from build123d import *

# Parameters (mm, degrees)
SKETCH1_W           = 30
SKETCH1_H           = 75
BOSS_EXTRUDE1_DEPTH = 12
CUT_EXTRUDE1_DEPTH  = 12
LPATTERN1_COUNT     = 3
LPATTERN1_PITCH     = 20
CUT_EXTRUDE2_DEPTH  = 30
BOSS_EXTRUDE2_DEPTH = 30
BOUNDARY1_START     = -45
BOUNDARY1_DEPTH     = 5
LPATTERN2_COUNT     = 3
LPATTERN2_PITCH     = 20


# Read off the part's stored shape, not the designer's step: Boundary1
with BuildPart() as part:
    # Sketch1 → Boss-Extrude1 (new body)
    with BuildSketch(Plane(origin=(0, 0, 0), x_dir=(1, 0, 0), z_dir=(0, 1, 0))):
        with Locations((15, 37.5)):
            Rectangle(SKETCH1_W, SKETCH1_H)
    extrude(amount=BOSS_EXTRUDE1_DEPTH)

    # Sketch3 → Cut-Extrude1 (cut)
    with BuildSketch(Plane(origin=(0, 0, 0), x_dir=(1, 0, 0), z_dir=(0, 1, 0))):
        Polygon((0, 5), (22.5, 12.5), (0, 20), align=None)
    cut_extrude1 = extrude(amount=CUT_EXTRUDE1_DEPTH, mode=Mode.SUBTRACT)

    # LPattern1: Cut-Extrude1 ×3
    with Locations(*[(0, 0, -i * LPATTERN1_PITCH) for i in range(1, LPATTERN1_COUNT)]):
        add(cut_extrude1, mode=Mode.SUBTRACT)

    # Sketch6 → Cut-Extrude2 (cut)
    with BuildSketch(Plane(origin=(0, 0, 0), x_dir=(0, 0, -1), z_dir=(1, 0, 0))):
        Polygon((60, 0), (75, 0), (75, 5.459553514), align=None)
    extrude(amount=CUT_EXTRUDE2_DEPTH, mode=Mode.SUBTRACT)

    # Sketch12 → Boss-Extrude2 (add)
    with BuildSketch(Plane.ZY):
        Polygon((-60, 12), (-75, 12), (-75, 17.459553514), align=None)
    extrude(amount=-BOSS_EXTRUDE2_DEPTH)

    # Boundary1 outline → Boundary1 (add)
    with BuildSketch(Plane.XY.offset(BOUNDARY1_START)):
        Polygon((25, 0), (25, -2), (30, 0), align=None)
    boundary1 = extrude(amount=BOUNDARY1_DEPTH)

    # LPattern2: Boundary1 ×3
    with Locations(*[(0, 0, i * LPATTERN2_PITCH) for i in range(1, LPATTERN2_COUNT)]):
        add(boundary1)


solid = part.part
Input: part model. Units: mm. Frame: model coordinates. A direction names the side the tool comes from. Give positions to 0.01 mm unless a question says otherwise; leave off trailing zeros. Loops run counter-clockwise (first coordinate to the right, second up) from the corner with the lowest first, then second, coordinate; pieces in that order, holes last. Notation, with made-up numbers: (11.5, 63) - (52.5, 63) arc R15 ccw to (52.5, 77) - close; hole circle Ø6 at (86.5, 77). An arc over 180 degrees is marked (long way). Use CSV: the item, a comma, the result in double quotes. Start each with the question number.
Item 1: Mould query, pull axis Z, two halves, no side actions, for faces 1 (the flat face through (27.5, -1, -2.5)), 2 (the flat face through (27, -1, -40)), 3 (the flat face through (27, -1, -45)). Classes: pulls with the +Z half, pulls with the -Z half, needs draft (parallel to the pull), parting line crosses it, or undercut.
Item 2: Section D-D on z = -35. Return loops of the section in (x, y).
Item 3: Section C-C on x = 21. Return loops of the section in (y, z), then the cut area to 3 significant figures.
Item 4: Reachability of faces 4 (the flat face through (11.1, 5.9, -28.7)), 5 (the flat face through (25, -1, -3)), 6 (the flat face through (27, -1, -25)) from +Z, -Z, +X, -X, +Y, -Y: full face, straight path, thin tool, end or side. Return the list, or none.
Item 5: Line query: line 1 (Z direction, x = 19, y = 8.5); line 2 (Z direction, x = 9.5, y = 7); line 3 (Y direction, x = 10, z = -26). Output: solid intervals per line, ascending.
Item 6: Contact query for flat-ended pins moving along their axis: P1, Ø12, axis at x = 9, z = -56, coming from the -Y side; P2, Ø1, axis at x = 26.5, y = 6.5, coming from the +Z side; P3, Ø12, axis at x = 27, z = -9, coming from the +Y side; P4, Ø1, axis at y = -1, z = -23, coming from the -X side. Output: stop coordinate, or through.
Item 7: Section A-A on x = 9.75. Return loops of the section in (y, z), then the cut area to 3 significant figures.
Item 8: Section B-B on y = 11.25. Return loops of the section in (x, z).
Ans:
1,face 1,"needs draft"
1,face 2,"undercut"
1,face 3,"pulls with the -Z half"
2,outline,"(15, 0) - (30, 0) - (30, 12) - (15, 12) - close"
3,outline,"(0, -60) - (5.46, -75) - (17.46, -75) - (12, -60) - (12, -53) - (0, -53) - close; (0, -52) - (12, -52) - (12, -33) - (0, -33) - close; (0, -32) - (12, -32) - (12, -13) - (0, -13) - close; (0, -12) - (12, -12) - (12, 0) - (0, 0) - close"
3,area,"864 mm2"
4,face 4,"-X, +Y, -Y"
4,face 5,"+Z, -Z, -X, -Y"
4,face 6,"+X, -X, -Y"
5,line 1,"z = -75 to -53.67, -51.33 to -33.67, -31.33 to -13.67, -11.33 to 0"
5,line 2,"z = -75 to -56.83, -48.17 to -36.83, -28.17 to -16.83, -8.17 to 0"
5,line 3,"y = 0 to 12"
6,P1,"stops at y = 0"
6,P2,"stops at z = 0"
6,P3,"stops at y = 12"
6,P4,"stops at x = 25"
7,outline,"(0, -60) - (5.46, -75) - (17.46, -75) - (12, -60) - (12, -56.75) - (0, -56.75) - close; (0, -48.25) - (12, -48.25) - (12, -36.75) - (0, -36.75) - close; (0, -28.25) - (12, -28.25) - (12, -16.75) - (0, -16.75) - close; (0, -8.25) - (12, -8.25) - (12, 0) - (0, 0) - close"
7,area,"594 mm2"
8,outline,"(0, -75) - (30, -75) - (30, 0) - (0, 0) - (0, -5) - (22.5, -12.5) - (0, -20) - (0, -25) - (22.5, -32.5) - (0, -40) - (0, -45) - (22.5, -52.5) - (0, -60) - close"
